Read the model definition and answer for the solid it produces. Units are mm, in the model's axes. Give positions to 0.01 mm unless a question says otherwise; leave off trailing zeros. Loops run counter-clockwise (first coordinate to the right, second up) from the corner with the lowest first, then second, coordinate; pieces in that order, holes last. Notation, with made-up numbers: (83, 88) - (99, 88) arc R19 cw to (99, 112) - close; hole circle Ø7 at (42.25, 59). An arc over 180 degrees is marked (long way). Write item = value, one per line.
```python
from build123d import *

# Parameters (mm, degrees)
F0_W     = 170
F0_H     = 342.370798
F1_DEPTH = 5
F2_R     = 1.5
F3_DEPTH = 5


with BuildPart() as f1:
    # F0 (on Top) → F1 (new body)
    with BuildSketch(Plane.XY):
        Rectangle(F0_W, F0_H)
    extrude(amount=F1_DEPTH)

    # F2 (on Top) → F3 (join)
    with BuildSketch(Plane.XY):
        with Locations((70, -166.185399)):
            Circle(F2_R)
        with Locations((-70, -166.185399)):
            Circle(F2_R)
        with Locations((70, 166.185399)):
            Circle(F2_R)
        with Locations((-70, 166.185399)):
            Circle(F2_R)
    extrude(amount=-F3_DEPTH)


solid = f1.part
```
1) A cutting plane is placed at A-A on y = 116. Determine the outline of the cut face in (x, z), then the cut area to 3 significant figures.
Output:
outline = (-85, 0) - (85, 0) - (85, 5) - (-85, 5) - close
area = 850 mm²
2) Find the intervals of material crossed by probe 1 along Z at (x, y) = (26, -155), in increasing order.
Output:
probe_1 = 0 to 5
3) This flat-tipped pin is pushed along its axis until it touches: P1, Ø10, axis at x = 13.5, y = 92.5, coming from the -Z side. Where does it stop, or does it pass through?
Output:
P1 = 0
4) A cutting plane is placed at B-B on x = 63. Determine the outline of the cut face in (y, z), then the cut area to 3 significant figures.
Output:
outline = (-171.19, 0) - (171.19, 0) - (171.19, 5) - (-171.19, 5) - close
area = 1,710 mm²
5) A cutting plane is placed at C-C on z = -3.25. Determine the outline of the cut face in (x, y).
Output:
outline = circle Ø3 at (-70, -166.19); circle Ø3 at (-70, 166.19); circle Ø3 at (70, -166.19); circle Ø3 at (70, 166.19)
